```python
from build123d import *

# Parameters (mm, degrees)
F0_W     = 30
F0_H     = 30
F1_DEPTH = 80
F2_W     = 30
F2_H     = 8.1
F3_DEPTH = 20
F4_R     = 8
F5_SIZE  = 2
F6_R     = 10
F7_DEPTH = 25
F8_SIZE  = 3


with BuildPart() as f1:
    # F0 (on Top) → F1 (new body)
    with BuildSketch(Plane.XY):
        Rectangle(F0_W, F0_H)
    extrude(amount=F1_DEPTH)

    # F2 (on face) → F3 (cut)
    with BuildSketch(Plane.YZ.offset(15)):
        with Locations((0, 14.05)):
            Rectangle(F2_W, F2_H)
    extrude(amount=-F3_DEPTH, mode=Mode.SUBTRACT)

    # F4
    f4_edges = [f1.edges().sort_by_distance(p)[0] for p in [
        (15, 0, 80),
        (-15, 0, 80),
    ]]
    fillet(f4_edges, radius=F4_R)

    # F5
    f5_edges = [f1.edges().sort_by_distance(p)[0] for p in [
        (15, 0, 18.1),
        (15, 0, 10),
    ]]
    chamfer(f5_edges, length=F5_SIZE)

    # F6 (on face) → F7 (join)
    with BuildSketch(Plane(origin=(0, 15, 0), x_dir=(-1, 0, 0), z_dir=(0, 1, 0))):
        with Locations((0, 65)):
            Circle(F6_R)
    extrude(amount=F7_DEPTH)

    # F8
    f8_edges = [f1.edges().sort_by_distance(p)[0] for p in [
        (10, 40, 65),
    ]]
    chamfer(f8_edges, length=F8_SIZE)


solid = f1.part
```
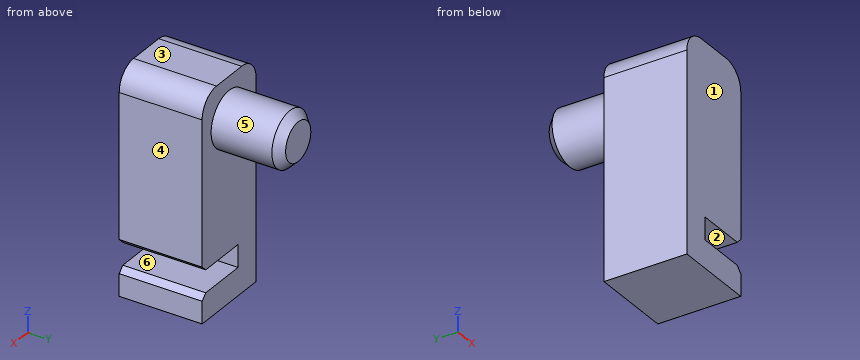
Input: part model. Units: mm. Frame: model coordinates. Face numbers are marked on the shaded views. A direction names the side the tool comes from. Give positions to 0.01 mm unless a question says otherwise; leave off trailing zeros. Order: outer loops, then holes, each group sorted by start corner. A loop starts at its lowest first (then second) coordinate and runs counter-clockwise, first axis right, second up. Notation, with made-up numbers: M 9,33 L 33,33 A33 ccw 33,62 Z; hole C -21,-18.5 d7. An arc over 180 degrees is marked long. Return JSON: item names as keys, results as strings.
Item 1: First-contact query: P1, Ø5, axis at x = -0.5, y = 20, coming from the -Z side; P2, Ø4, axis at y = 2.5, z = 15.5, coming from the +X side; P3, Ø5, axis at y = 26, z = 63, coming from the -X side. Flat tips, straight axial feed; report the tip coordinate or a pass-through.
Solutions:
{"P1": "z = 55", "P2": "x = -5", "P3": "x = -10"}
Item 2: Access query for the marked faces 4, 5 and 6. Directions: +Z, -Z, +X, -X, +Y, -Y. A direction counts if a zero-diameter tool reaches every point of the face in a straight line with its end or side. Return the directions, or none.
Solutions:
{"face 4": "+Z, -Z, +X, +Y, -Y", "face 5": "+Y", "face 6": "+X, +Y, -Y"}
Item 3: Ray query, probe 1 along Z at (x, y) = (-0.5, 3); probe 2 along Y at (x, z) = (9, 31); probe 3 along Z at (x, y) = (-7.5, 4). Return the intervals inside material, ascending.
Solutions:
{"probe 1": "0 to 10, 18.1 to 80", "probe 2": "-15 to 15", "probe 3": "0 to 79.98"}
Item 4: Cut plane C-C (z = 65). Return loops of the section in (x, y).
Solutions:
{"outline": "M -15,-15 L 15,-15 L 15,15 L 10,15 L 10,37 L 7,40 L -7,40 L -10,37 L -10,15 L -15,15 Z"}
Item 5: Cut plane D-D (y = 33.5). Return loops of the section in (x, z), then the cut area to 3 significant figures.
Solutions:
{"outline": "C 0,65 d20", "area": "314 mm^2"}
Item 6: Cut plane A-A (x = 0). Return loops of the section in (y, z), then the cut area to 3 significant figures.
Solutions:
{"outline": "M -15,0 L 15,0 L 15,10 L -15,10 Z; M -15,18.1 L 15,18.1 L 15,55 L 37,55 L 40,58 L 40,72 L 37,75 L 15,75 L 15,80 L -15,80 Z", "area": "2,650 mm^2"}
Item 7: Pull-direction query (Z, two-part tool) for the marked faces 1, 2 and 3; classes: +Z half, -Z half, draft (parallel to the pull), parting line (faces both ways), or undercut.
Solutions:
{"face 1": "draft", "face 2": "undercut", "face 3": "+Z half"}
Item 8: Cut plane B-B (y = 1.5). Return loops of the section in (x, z).
Solutions:
{"outline": "M -15,0 L 15,0 L 15,8 L 13,10 L -5,10 L -5,18.1 L 13,18.1 L 15,20.1 L 15,72 A8 ccw 7,80 L -7,80 A8 ccw -15,72 Z"}
